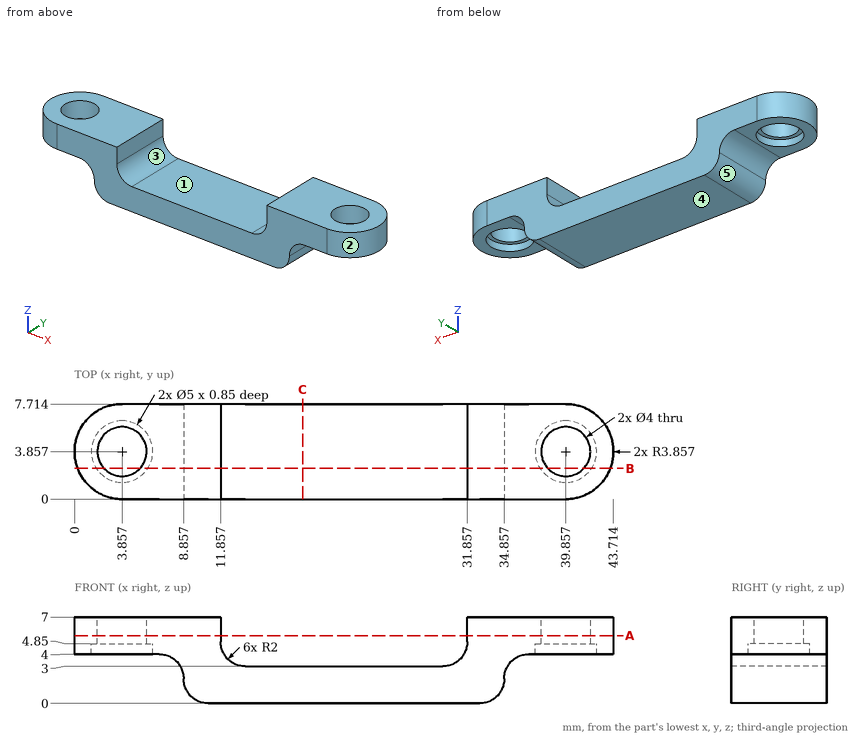
Geometry: see drawing. Coordinates: mm, zero at the bounding-box minimum. A direction names the side the tool comes from. Give positions to 0.01 mm unless a question says otherwise; leave off trailing zeros. Loops run counter-clockwise (first coordinate to the right, second up) from the corner with the lowest first, then second, coordinate; pieces in that order, holes last. Notation, with made-up numbers: (73, 35) - (89, 35) arc R13 cw to (89, 53) - close; hole circle Ø8 at (87.25, 56.5). An arc over 180 degrees is marked (long way). Use CSV: the item, a comma, the result in double quotes. Start each with the question number.
1. Pin query (flat end, axial travel): pin 1 (1.6 mm diameter, centred on y = 4, z = 6, fed in from +X); pin 2 (1.5 mm diameter, centred on y = 5, z = 2, fed in from -X); pin 3 (3 mm diameter, centred on x = 39.86, y = 3.86, fed in from +Z); pin 4 (2.5 mm diameter, centred on x = 4.5, y = 2.5, fed in from -Z). Return the tip coordinate at first contact, or that it passes through.
2. Section B-B (y = 2.5). Count the separate pieces of the cut face and the enclosed holes in it, then the cut area to 3 significant figures.
3. Section C-C (x = 18.5). Output: boundary loops of the cut face in (y, z) (1 decimal).
4. Ray query, L1, parallel to Z at x = 37, y = 0.5; L2, parallel to Y at x = 5.5, z = 5.75 (1 decimal); L3, parallel to Z at x = 14.5, y = 1.25. Return the intervals inside material, ascending.
5. Draft query along X for the marked faces 3, 4 and 5. Return one class per face: +X half, -X half, draft (parallel to the pull), parting line (faces both ways), or undercut.
6. Section A-A (z = 5.5). Output: boundary loops of the cut face in (x, y) (1 decimal).
7. Reachability of the marked faces 1 and 2 from +Z, -Z, +X, -X, +Y, -Y: full face, straight path, thin tool, end or side. Return the list, or none.
Response:
1,pin 1,"x = 43.71"
1,pin 2,"x = 8.71"
1,pin 3,"through"
1,pin 4,"z = 4"
2,separate pieces,"3"
2,enclosed holes,"0"
2,area,"136 mm²"
3,outline,"(0, 0) - (7.7, 0) - (7.7, 3) - (0, 3) - close"
4,L1,"4 to 7"
4,L2,"0 to 2.7, 5 to 7.7"
4,L3,"0 to 3"
5,face 3,"undercut"
5,face 4,"draft"
5,face 5,"-X half"
6,outline,"(3.9, 0) - (11.9, 0) - (11.9, 7.7) - (3.9, 7.7) arc R3.9 ccw to start; (31.9, 0) - (39.9, 0) arc R3.9 ccw to (39.9, 7.7) - (31.9, 7.7) - close; hole circle Ø4 at (3.9, 3.9); hole circle Ø4 at (39.9, 3.9)"
7,face 1,"+Z, +Y, -Y"
7,face 2,"+Z, -Z, +X"
